from build123d import *

# Parameters (mm, degrees)
SKETCH1_W                      = 44
SKETCH1_H                      = 40
SKETCH1_R                      = 4
BOSS_EXTRUDE1_DEPTH            = 14
CUT_EXTRUDE1_REACH             = 18.442
SKETCH2_W                      = 16
SKETCH2_H                      = 7.114924263
CUT_EXTRUDE1_DIRECTION_2_REACH = 25.558


with BuildPart() as part:
    # Sketch1 → Boss-Extrude1 (new body)
    with BuildSketch(Plane(origin=(0, 0, 0), x_dir=(1, 0, 0), z_dir=(0, 1, 0))):
        with Locations((-0.188936111, 3.557633072)):
            Rectangle(SKETCH1_W, SKETCH1_H)
        with Locations((14.811063889, -8.442366928)):
            Circle(SKETCH1_R, mode=Mode.SUBTRACT)
        with Locations((14.811063889, 15.557633072)):
            Circle(SKETCH1_R, mode=Mode.SUBTRACT)
        with Locations((-15.188936111, 15.557633072)):
            Circle(SKETCH1_R, mode=Mode.SUBTRACT)
        with Locations((-15.188936111, -8.442366928)):
            Circle(SKETCH1_R, mode=Mode.SUBTRACT)
    extrude(amount=BOSS_EXTRUDE1_DEPTH)

    # Cut-Extrude1: up to this face of the body (flat: up to its plane)
    cut_extrude1_end = Plane(part.part.faces().sort_by_distance((-0.188936111, 7, 16.442366928))[0])
    # Sketch2 → Cut-Extrude1 (cut, up to the picked face)
    with BuildSketch(Plane.XY, mode=Mode.PRIVATE) as cut_extrude1_sk1:
        with Locations((0, 1.442537868)):
            Rectangle(SKETCH2_W, SKETCH2_H)
    cut_extrude1_tool1 = split(extrude(cut_extrude1_sk1.sketch, amount=CUT_EXTRUDE1_REACH, mode=Mode.PRIVATE), bisect_by=cut_extrude1_end, keep=Keep.BOTH, mode=Mode.PRIVATE)
    add(cut_extrude1_tool1.solids().sort_by_distance((0, 1.442538, 0))[0], mode=Mode.SUBTRACT)

    # Cut-Extrude1 direction 2: up to this face of the body (flat: up to its plane)
    cut_extrude1_direction_2_end = Plane(part.part.faces().sort_by_distance((-0.188936111, 7, -23.557633072))[0])
    # Sketch2 → Cut-Extrude1 direction 2 (cut, up to the picked face)
    with BuildSketch(Plane.XY, mode=Mode.PRIVATE) as cut_extrude1_direction_2_sk1:
        with Locations((0, 1.442537868)):
            Rectangle(SKETCH2_W, SKETCH2_H)
    cut_extrude1_direction_2_tool1 = split(extrude(cut_extrude1_direction_2_sk1.sketch, amount=-CUT_EXTRUDE1_DIRECTION_2_REACH, mode=Mode.PRIVATE), bisect_by=cut_extrude1_direction_2_end, keep=Keep.BOTH, mode=Mode.PRIVATE)
    add(cut_extrude1_direction_2_tool1.solids().sort_by_distance((0, 1.442538, 0))[0], mode=Mode.SUBTRACT)


solid = part.part
Model file for the job. Use its own axes, mm. A direction names the side the tool comes from. Round coordinates to 2 decimals unless told otherwise and drop trailing zeros. Order: outer loops, then holes, each group sorted by start corner. A loop starts at its lowest first (then second) coordinate and runs counter-clockwise, first axis right, second up.
(1) Band-saw the part on A-A (y = 3). List the corners of the cut face in (x, z), then the cut area to 3 significant figures.
(2) Band-saw the part on D-D (y = 8.5). List the corners of the cut face in (x, z), then the cut area to 3 significant figures.
(3) 3-axis set-ups, long thin cutter, end or side, ignore diameter. For faces 5 (the face through (-22.189, 7, -3)), 6 (the face through (0, 5, -4)): which of +Z, -Z, +X, -X, +Y, -Y reach the whole face in a straight line?
(4) Drill centre lines: line 1 (Z direction, x = -15, y = 9); line 2 (X direction, y = 11, z = 8); line 3 (X direction, y = 2, z = -2). Where is each one in solid material? Low to high.
(5) Pin check, flat tips, straight feed: pin 1 (10.5 mm diameter, centred on x = -15.19, z = 8.44, fed in from -Y); pin 2 (4 mm diameter, centred on x = 15.5, z = 9, fed in from -Y); pin 3 (8 mm diameter, centred on x = -3.5, z = -0.5, fed in from -Y). Stop position of each tip, or through.
(6) Pull direction X, two halves, no side cores. Call faces 1 (the face through (21.811, 7, -3)), 2 (the face through (0, 14, -4)), 3 (the face through (10.815, 6.902, 8.266)), 4 (the face through (10.815, 6.902, -15.734)): released by +X, released by -X, zero draft, split by the parting line, or undercut.
(7) Band-saw the part on C-C (z = -15). List the corners of the cut face in (x, y), then the cut area to 3 significant figures.
(8) Band-saw the part on B-B (z = 0.5). List the corners of the cut face in (x, y), then the cut area to 3 significant figures.
Verdict:
1. outline: (-22.19, -23.56) - (-8, -23.56) - (-8, 16.44) - (-22.19, 16.44) - close; (8, -23.56) - (21.81, -23.56) - (21.81, 16.44) - (8, 16.44) - close; hole circle Ø8 at (-15.19, -15.56); hole circle Ø8 at (-15.19, 8.44); hole circle Ø8 at (14.81, -15.56); hole circle Ø8 at (14.81, 8.44)
1. area: 919 mm2
2. outline: (-22.19, -23.56) - (21.81, -23.56) - (21.81, 16.44) - (-22.19, 16.44) - close; hole circle Ø8 at (-15.19, -15.56); hole circle Ø8 at (-15.19, 8.44); hole circle Ø8 at (14.81, -15.56); hole circle Ø8 at (14.81, 8.44)
2. area: 1,560 mm2
3. face 5: +Z, -Z, -X, +Y, -Y
3. face 6: +Z, -Z, -Y
4. line 1: z = -23.56 to -19.55, -11.56 to 4.45, 12.44 to 16.44
4. line 2: x = -22.19 to -19.16, -11.21 to 10.84, 18.79 to 21.81
4. line 3: x = -22.19 to -8, 8 to 21.81
5. pin 1: stops at y = 0
5. pin 2: passes through
5. pin 3: stops at y = 5
6. face 1: released by +X
6. face 2: zero draft
6. face 3: undercut
6. face 4: undercut
7. outline: (-22.19, 0) - (-19.15, 0) - (-19.15, 14) - (-22.19, 14) - close; (-11.23, 0) - (-8, 0) - (-8, 5) - (8, 5) - (8, 0) - (10.85, 0) - (10.85, 14) - (-11.23, 14) - close; (18.77, 0) - (21.81, 0) - (21.81, 14) - (18.77, 14) - close
7. area: 314 mm2
8. outline: (-22.19, 0) - (-8, 0) - (-8, 5) - (8, 5) - (8, 0) - (21.81, 0) - (21.81, 14) - (-22.19, 14) - close
8. area: 536 mm2
